Autodesk Inventor part; units mm, degrees
ref_plane "YZ Plane" through (0, 0, 0) normal (1, 0, 0) x (0, 1, 0)
ref_plane "XZ Plane" through (0, 0, 0) normal (0, 1, 0) x (-1, 0, 0)
ref_plane "XY Plane" through (0, 0, 0) normal (0, 0, 1) x (1, 0, 0)
sketch "Sketch1" plane through (0, 0, 0) normal (0, 1, 0) x (-1, 0, 0)
  line L0 (0, 0) -> (36.25, 0) construction
  line L1 (36.25, 0) -> (36.25, 31.6619)
  line L2 (36.0718, 34.3261) -> (35.1129, 41.4603)
  line L3 (34.1532, 42.3266) -> (0, 43.4)
  line L4 (0, 43.4) -> (0, 0) construction
  arc A0 (35.1129, 41.4603) -> (34.1532, 42.3266) centre (34.1218, 41.3271) ccw
  arc A1 (36.25, 31.6619) -> (36.0718, 34.3261) centre (16.25, 31.6619) ccw
  line L5 (36.25, 0) -> (36.25, -31.6619)
  line L6 (36.0718, -34.3261) -> (35.1129, -41.4603)
  line L7 (34.1532, -42.3266) -> (0, -43.4)
  arc A2 (34.1532, -42.3266) -> (35.1129, -41.4603) centre (34.1218, -41.3271) ccw
  arc A3 (36.0718, -34.3261) -> (36.25, -31.6619) centre (16.25, -31.6619) ccw
  line L8 (-36.25, 0) -> (-36.25, 31.6619)
  line L9 (-36.0718, 34.3261) -> (-35.1129, 41.4603)
  line L10 (-34.1532, 42.3266) -> (0, 43.4)
  arc A4 (-34.1532, 42.3266) -> (-35.1129, 41.4603) centre (-34.1218, 41.3271) ccw
  arc A5 (-36.0718, 34.3261) -> (-36.25, 31.6619) centre (-16.25, 31.6619) ccw
  line L11 (-36.0718, -34.3261) -> (-35.1129, -41.4603)
  arc A6 (-35.1129, -41.4603) -> (-34.1532, -42.3266) centre (-34.1218, -41.3271) ccw
  arc A7 (-36.25, -31.6619) -> (-36.0718, -34.3261) centre (-16.25, -31.6619) ccw
  line L12 (-36.25, 0) -> (-36.25, -31.6619)
  line L13 (-34.1532, -42.3266) -> (0, -43.4)
  point P0 (36.25, 33)
  point P1 (35, 42.3)
  point P2 (36.25, -33)
  point P3 (35, -42.3)
  point P4 (-36.25, 33)
  point P5 (-35, 42.3)
  point P6 (-36.25, -33)
  point P7 (-35, -42.3)
  dimension "d2" = 36.25
  dimension "d3" = 43.4
  dimension "d6" = 33
  dimension "d7" = 9.3
  dimension "d8" = 35
  dimension "d9" = 1
  dimension "d10" = 20
extrude "Extrusion1" add sketch "Sketch1" along normal blind 1.7
properties part number "End"
Model file for the job. Use its own axes, mm. Coordinates: 2 decimals unless noted, no trailing zeros. Write each loop counter-clockwise with the first axis right and the second up, starting at its lowest first coordinate (ties: lowest second). Pieces come first, ordered by that corner, then holes. Notation, with made-up numbers: (79.25, 29.5) - (106.25, 29.5) arc R30 ccw to (106.25, 60.5) - close; hole circle Ø11 at (53.5, -19.75). An arc over 180 degrees is marked (long way). One line per item, written item: value. Start each with the question number.
1. Probe line 1 (Z direction, x = -0.5, y = 0.35); line 2 (X direction, y = 0.85, z = 34.5); line 3 (X direction, y = 1.3, z = -38). List the from-to ranges inside material, lowest first. Write a range as from..to.
2. Slice it at A-A (y = 0.9). Write the cut outline in (x, z), plus the area to 3 significant figures.
3. Slice it at B-B (x = -29). Write the cut outline in (y, z).
Answers below:
1. line 1: z = -43.38..43.38
1. line 2: x = -36.05..36.05
1. line 3: x = -35.58..35.58
2. outline: (-36.25, -31.66) arc R19.99 ccw to (-36.07, -34.33) - (-35.11, -41.46) arc R1 ccw to (-34.15, -42.33) - (0, -43.4) - (34.15, -42.33) arc R1 ccw to (35.11, -41.46) - (36.07, -34.33) arc R20.01 ccw to (36.25, -31.66) - (36.25, 31.66) arc R19.99 ccw to (36.07, 34.33) - (35.11, 41.46) arc R1 ccw to (34.15, 42.33) - (0, 43.4) - (-34.15, 42.33) arc R1 ccw to (-35.11, 41.46) - (-36.07, 34.33) arc R20.01 ccw to (-36.25, 31.66) - close
2. area: 6,190 mm^2
3. outline: (0, -42.49) - (1.7, -42.49) - (1.7, 42.49) - (0, 42.49) - close
